```python
from build123d import *

# Parameters (mm, degrees)
SKETCH6_W                      = 43.1
SKETCH6_H                      = 48.18
SKETCH6_R                      = 2.5
BASE_FLANGE2_DEPTH             = 2
EDGE_FLANGE1_STRIP_W           = 9.4732
EDGE_FLANGE1_STRIP_H           = 2
EDGE_FLANGE1_STRIP_CUT_DEPTH   = 48.18
EDGE_FLANGE1_STRIP_2_W         = 9.4732
EDGE_FLANGE1_STRIP_2_H         = 2
EDGE_FLANGE1_STRIP_CUT_2_DEPTH = 48.18
EDGE_FLANGE1_DEPTH             = 48.18
EDGE_FLANGE1_BEND_DEPTH        = 48.18
EDGE_FLANGE3_DEPTH             = 43.1
EDGE_FLANGE3_2_DEPTH           = 2.7366
EDGE_FLANGE3_START             = 40.3634
EDGE_FLANGE3_3_DEPTH           = 2.7366
EDGE_FLANGE3_START_2           = -7.2634
EDGE_FLANGE3_4_OUTLINE_W       = 2
EDGE_FLANGE3_4_OUTLINE_H       = 11.9634
EDGE_FLANGE3_4_DEPTH           = 57.6268
EDGE_FLANGE3_START_3           = 2.7366
EDGE_FLANGE3_5_DEPTH           = 37.6268
FILLET3_R                      = 7
CUT_EXTRUDE1_REACH             = 74.599
SKETCH21_R                     = 2.1
FILLET4_R                      = 5


# Read off the part's stored shape, not the designer's step: Edge-Flange3
# Sheet-metal steps are written as plain solids
with BuildPart() as part:
    # Sketch6 → Base-Flange2 (new body)
    with BuildSketch(Plane.XY):
        with Locations((21.55, 24.09)):
            Rectangle(SKETCH6_W, SKETCH6_H)
        with Locations((31.23, 6.16)):
            Circle(SKETCH6_R, mode=Mode.SUBTRACT)
        with Locations((11.87, 6.16)):
            Circle(SKETCH6_R, mode=Mode.SUBTRACT)
        with Locations((11.87, 42.83)):
            Circle(SKETCH6_R, mode=Mode.SUBTRACT)
        with Locations((31.23, 42.83)):
            Circle(SKETCH6_R, mode=Mode.SUBTRACT)
    extrude(amount=-BASE_FLANGE2_DEPTH)

    # Edge-Flange1 strip (across the edge) → Edge-Flange1 strip cut (cut)
    with BuildSketch(Plane.XZ.offset(-48.18)):
        with Locations((-2, -1)):
            Rectangle(EDGE_FLANGE1_STRIP_W, EDGE_FLANGE1_STRIP_H)
    extrude(amount=EDGE_FLANGE1_STRIP_CUT_DEPTH, mode=Mode.SUBTRACT)

    # Edge-Flange1 strip 2 (across the edge) → Edge-Flange1 strip cut 2 (cut)
    with BuildSketch(Plane(origin=(43.1, 0, 0), x_dir=(-1, 0, 0), z_dir=(0, 1, 0))):
        with Locations((-2, -1)):
            Rectangle(EDGE_FLANGE1_STRIP_2_W, EDGE_FLANGE1_STRIP_2_H)
    extrude(amount=EDGE_FLANGE1_STRIP_CUT_2_DEPTH, mode=Mode.SUBTRACT)

    # Edge-Flange1 section (across the edge) → Edge-Flange1 (add)
    with BuildSketch(Plane.XZ.offset(-48.18)):
        with BuildLine():
            Line((0, 0.7366), (0, 8.05))
            Line((0, 8.05), (2, 8.05))
            Line((2, 8.05), (2, 0.7366))
            ThreePointArc((2, 0.7366), (2.215745145, 0.215745145), (2.7366, 0))
            Line((2.7366, 0), (2.7366, -2))
            ThreePointArc((2.7366, -2), (0.801531583, -1.198468417), (0, 0.7366))
        make_face()
    extrude(amount=EDGE_FLANGE1_DEPTH)

    # Edge-Flange1 section 2 (across the edge) → Edge-Flange1 bend (add)
    with BuildSketch(Plane(origin=(43.1, 0, 0), x_dir=(-1, 0, 0), z_dir=(0, 1, 0))):
        with BuildLine():
            Line((0, 0.7366), (0, 8.05))
            Line((0, 8.05), (2, 8.05))
            Line((2, 8.05), (2, 0.7366))
            ThreePointArc((2, 0.7366), (2.215745145, 0.215745145), (2.7366, 0))
            Line((2.7366, 0), (2.7366, -2))
            ThreePointArc((2.7366, -2), (0.801531583, -1.198468417), (0, 0.7366))
        make_face()
    extrude(amount=EDGE_FLANGE1_BEND_DEPTH)

    # Edge-Flange3 outline → Edge-Flange3 (cut)
    with BuildSketch(Plane.YZ):
        with BuildLine():
            Line((48.18, 0.7366), (47.4434, 0.7366))
            Line((47.4434, 0.7366), (47.4434, 0))
            ThreePointArc((47.4434, 0), (47.815145906, -0.025366971), (48.18, -0.100997602))
            Line((48.18, -0.100997602), (48.18, 0.7366))
        make_face()
    extrude(amount=EDGE_FLANGE3_DEPTH, mode=Mode.SUBTRACT)

    # Edge-Flange3 2 outline → Edge-Flange3 2 (cut)
    with BuildSketch(Plane.YZ):
        with BuildLine():
            ThreePointArc((48.18, -0.100997602), (47.815145906, -0.025366971), (47.4434, 0))
            Line((47.4434, 0), (47.4434, -2))
            ThreePointArc((47.4434, -2), (47.964254855, -2.215745145), (48.18, -2.7366))
            Line((48.18, -2.7366), (50.18, -2.7366))
            ThreePointArc((50.18, -2.7366), (49.623395312, -1.082332791), (48.18, -0.100997602))
        make_face()
    extrude(amount=EDGE_FLANGE3_2_DEPTH, mode=Mode.SUBTRACT)

    # Edge-Flange3 3 outline → Edge-Flange3 3 (cut)
    with BuildSketch(Plane.YZ.offset(EDGE_FLANGE3_START)):
        with BuildLine():
            ThreePointArc((48.18, -0.100997602), (47.815145906, -0.025366971), (47.4434, 0))
            Line((47.4434, 0), (47.4434, -2))
            ThreePointArc((47.4434, -2), (47.964254855, -2.215745145), (48.18, -2.7366))
            Line((48.18, -2.7366), (50.18, -2.7366))
            ThreePointArc((50.18, -2.7366), (49.623395312, -1.082332791), (48.18, -0.100997602))
        make_face()
    extrude(amount=EDGE_FLANGE3_3_DEPTH, mode=Mode.SUBTRACT)



with BuildPart() as body_2:
    # Edge-Flange3 4 outline → Edge-Flange3 4 (new body)
    with BuildSketch(Plane.YZ.offset(EDGE_FLANGE3_START_2)):
        with Locations((49.18, -8.7183)):
            Rectangle(EDGE_FLANGE3_4_OUTLINE_W, EDGE_FLANGE3_4_OUTLINE_H)
    extrude(amount=EDGE_FLANGE3_4_DEPTH)


with BuildPart() as part_1:
    add(part.part)

    add(body_2.part)  # Edge-Flange3 5 merges body 2
    # Edge-Flange3 5 outline → Edge-Flange3 5 (add)
    with BuildSketch(Plane.YZ.offset(EDGE_FLANGE3_START_3)):
        with BuildLine():
            ThreePointArc((48.18, -0.100997602), (47.815145906, -0.025366971), (47.4434, 0))
            Line((47.4434, 0), (47.4434, -2))
            ThreePointArc((47.4434, -2), (47.964254855, -2.215745145), (48.18, -2.7366))
            Line((48.18, -2.7366), (50.18, -2.7366))
            ThreePointArc((50.18, -2.7366), (49.623395312, -1.082332791), (48.18, -0.100997602))
        make_face()
    extrude(amount=EDGE_FLANGE3_5_DEPTH)

    # Fillet3
    fillet3_edges = [part_1.edges().sort_by_distance(p)[0] for p in [
        (-7.2634, 49.18, -14.7),
        (50.3634, 49.18, -14.7),
        (1, 48.18, 8.05),
        (1, 0, 8.05),
        (42.1, 0, 8.05),
        (42.1, 48.18, 8.05),
    ]]
    fillet(fillet3_edges, radius=FILLET3_R)

    # Sketch21 → Cut-Extrude1 (cut, up to next)
    with BuildSketch(Plane(origin=(0, 50.18, 0), x_dir=(1, 0, 0), z_dir=(0, 1, 0)), mode=Mode.PRIVATE) as cut_extrude1_sk1:
        with Locations(Location((1.55, 8.322080502, 0), (0, 0, 270))):
            Circle(SKETCH21_R)
    cut_extrude1_tool1 = extrude(cut_extrude1_sk1.sketch, amount=-CUT_EXTRUDE1_REACH, mode=Mode.PRIVATE) & part_1.part
    # Sketch21 → Cut-Extrude1 (cut, up to next)
    with BuildSketch(Plane(origin=(0, 50.18, 0), x_dir=(1, 0, 0), z_dir=(0, 1, 0)), mode=Mode.PRIVATE) as cut_extrude1_sk2:
        with Locations(Location((41.55, 8.322080502, 0), (0, 0, 270))):
            Circle(SKETCH21_R)
    cut_extrude1_tool2 = extrude(cut_extrude1_sk2.sketch, amount=-CUT_EXTRUDE1_REACH, mode=Mode.PRIVATE) & part_1.part
    add(cut_extrude1_tool1.solids().sort_by_distance((1.55, 50.18, -8.322081))[0], mode=Mode.SUBTRACT)
    add(cut_extrude1_tool2.solids().sort_by_distance((41.55, 50.18, -8.322081))[0], mode=Mode.SUBTRACT)

    # Fillet4
    fillet4_edges = [part_1.edges().sort_by_distance(p)[0] for p in [
        (50.3634, 49.18, -2.7366),
        (-7.2634, 49.18, -2.7366),
    ]]
    fillet(fillet4_edges, radius=FILLET4_R)


solid = part_1.part
```
Geometry: final body of the model. Coordinates: model frame, mm. A direction names the side the tool comes from. Coordinates: 2 decimals unless noted, no trailing zeros. Loops run counter-clockwise (first coordinate to the right, second up) from the corner with the lowest first, then second, coordinate; pieces in that order, holes last. Notation, with made-up numbers: (83.25, 46.5) -> (124.25, 46.5) arc R15 cw to (124.25, 72.5) -> close; hole circle Ø5 at (-1.5, -33). An arc over 180 degrees is marked (long way). Use a Markdown table: item, result. Add a question column.
(1) Mould query, pull axis X, two halves, no side actions, for faces 5 (the cylindrical face through (42.277, 23.39, -1.22)), 6 (the cylindrical face through (43.63, 49.19, -8.6)), 7 (the cylindrical face through (1.01, 2, 5.95)). Classes: pulls with the +X half, pulls with the -X half, needs draft (parallel to the pull), parting line crosses it, or undercut.
(2) Section query B-B, the plane y = 42.83. Return loops of the section in (x, z), plus the area to 3 significant figures.
(3) Section query A-A, the plane x = 11.87. Return loops of the section in (y, z).
(4) Access query for faces 1 (the flat face through (0, 49, -2.737)), 2 (the flat face through (40.363, 49, -1)), 3 (the flat face through (21, 24, 0)), 4 (the flat face through (42, 47.443, -1)). Directions: +Z, -Z, +X, -X, +Y, -Y. A direction counts if a zero-diameter tool reaches every point of the face in a straight line with its end or side. Return the directions, or none.
(5) Line query: line 1 along Y through (x, z) = (11.87, -1.3); line 2 along X through (y, z) = (39, 0.75); line 3 along Z through (x, y) = (5, 38.5). Output: solid intervals per line, ascending.
(6) Section query D-D, the plane x = 26. Return loops of the section in (y, z), plus the area to 3 significant figures.
(7) Pin query (flat end, axial travel): pin 1 Ø11.5 at (x, y) = (30.5, 12) entering from -Z; pin 2 Ø3.5 at (y, z) = (18, 3.5) entering from +X; pin 3 Ø6.5 at (x, y) = (31.23, 6.16) entering from +Z. Return the tip coordinate at first contact, or that it passes through.
(8) Section query C-C, the plane z = 2.5. Return loops of the section in (x, y), plus the area to 3 significant figures.
Answer:
| question | item | result |
|---|---|---|
| 1 | face 5 | pulls with the +X half |
| 1 | face 6 | undercut |
| 1 | face 7 | needs draft |
| 2 | outline | (0, 0.74) arc R2.74 ccw to (2.74, -2) -> (9.37, -2) -> (9.37, 0) -> (2.74, 0) arc R0.74 cw to (2, 0.74) -> (2, 7.85) -> (0, 7.85) -> close; (14.37, -2) -> (28.73, -2) -> (28.73, 0) -> (14.37, 0) -> close; (33.73, -2) -> (40.36, -2) arc R2.74 ccw to (43.1, 0.74) -> (43.1, 7.85) -> (41.1, 7.85) -> (41.1, 0.74) arc R0.74 cw to (40.36, 0) -> (33.73, 0) -> close |
| 2 | area | 94.6 mm^2 |
| 3 | outline | (0, -2) -> (3.66, -2) -> (3.66, 0) -> (0, 0) -> close; (8.66, -2) -> (40.33, -2) -> (40.33, 0) -> (8.66, 0) -> close; (45.33, -2) -> (47.44, -2) arc R0.74 cw to (48.18, -2.74) -> (48.18, -14.7) -> (50.18, -14.7) -> (50.18, -2.74) arc R2.74 ccw to (47.44, 0) -> (45.33, 0) -> close |
| 4 | face 1 | +Z, -X, +Y, -Y |
| 4 | face 2 | +Z, +X, +Y |
| 4 | face 3 | +Z, +Y, -Y |
| 4 | face 4 | -Z, +X, +Y |
| 5 | line 1 | y = 0 to 3.66, 8.66 to 40.33, 45.33 to 49.77 |
| 5 | line 2 | x = 0 to 2, 41.1 to 43.1 |
| 5 | line 3 | z = -2 to 0 |
| 6 | outline | (0, -2) -> (47.44, -2) arc R0.74 cw to (48.18, -2.74) -> (48.18, -14.7) -> (50.18, -14.7) -> (50.18, -2.74) arc R2.74 ccw to (47.44, 0) -> (0, 0) -> close |
| 6 | area | 124 mm^2 |
| 7 | pin 1 | stops at z = -2 |
| 7 | pin 2 | stops at x = 43.1 |
| 7 | pin 3 | stops at z = 0 |
| 8 | outline | (0, 0.15) -> (2, 0.15) -> (2, 48.03) -> (0, 48.03) -> close; (41.1, 0.15) -> (43.1, 0.15) -> (43.1, 48.03) -> (41.1, 48.03) -> close |
| 8 | area | 192 mm^2 |
